Could you check a few things on this model? Use its own coordinates, in mm. Round coordinates to 2 decimals unless told otherwise and drop trailing zeros. Order: outer loops, then holes, each group sorted by start corner. A loop starts at its lowest first (then second) coordinate and runs counter-clockwise, first axis right, second up. Notation, with made-up numbers: (-32.5, 7) -> (19.5, 7) arc R30 cw to (19.5, 37) -> close; hole circle Ø10 at (58, 42.5). An arc over 180 degrees is marked (long way). One line per question, with ' | ' between items.
```python
from build123d import *

# Parameters (mm, degrees)
F0_W     = 32.5
F0_H     = 4
F0_W_2   = 15
F1_DEPTH = 4


with BuildPart() as f1:
    # F0 (on Top) → F1 (new body)
    with BuildSketch(Plane.XY):
        Polygon((0, -16), (0, 0), (-148, 0), (-148, -16), (-148, -20), (-148, -36), (0, -36), (0, -20), align=None)
        with Locations((-127.75, -18)):
            Rectangle(F0_W, F0_H, mode=Mode.SUBTRACT)
        with Locations((-89, -18)):
            Rectangle(F0_W_2, F0_H, mode=Mode.SUBTRACT)
        with Locations((-59, -18)):
            Rectangle(F0_W_2, F0_H, mode=Mode.SUBTRACT)
        with Locations((-20.25, -18)):
            Rectangle(F0_W, F0_H, mode=Mode.SUBTRACT)
    extrude(amount=F1_DEPTH)


solid = f1.part
```
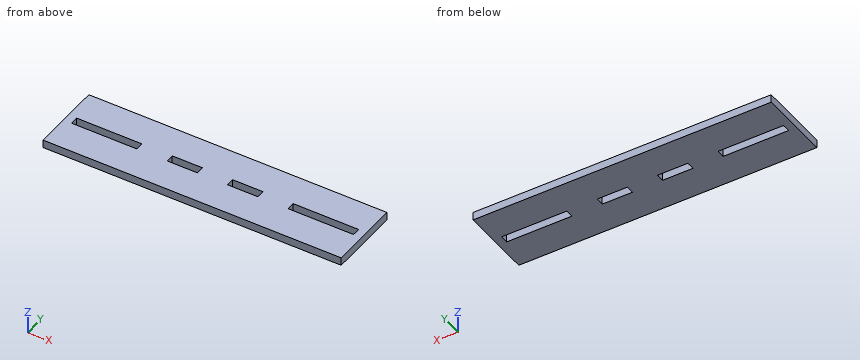
1. I need wall thicknesses on probe 1 along Y at (x, z) = (-131, 2.8); probe 2 along X at (y, z) = (-18, 1.5). Which ranges of each line are inside material? Lowest first, please.
From the geometry:
probe 1: y = -36 to -20, -16 to 0 | probe 2: x = -148 to -144, -111.5 to -96.5, -81.5 to -66.5, -51.5 to -36.5, -4 to 0
2. I want a section at B-B on y = -17.5. List the corners of the cut face in (x, z) for me, and give its area (3 significant figures).
From the geometry:
outline: (-148, 0) -> (-144, 0) -> (-144, 4) -> (-148, 4) -> close; (-111.5, 0) -> (-96.5, 0) -> (-96.5, 4) -> (-111.5, 4) -> close; (-81.5, 0) -> (-66.5, 0) -> (-66.5, 4) -> (-81.5, 4) -> close; (-51.5, 0) -> (-36.5, 0) -> (-36.5, 4) -> (-51.5, 4) -> close; (-4, 0) -> (0, 0) -> (0, 4) -> (-4, 4) -> close | area: 212 mm²
3. I want a section at A-A on x = -132. List the corners of the cut face in (y, z) for me.
From the geometry:
outline: (-36, 0) -> (-20, 0) -> (-20, 4) -> (-36, 4) -> close; (-16, 0) -> (0, 0) -> (0, 4) -> (-16, 4) -> close
4. I want a section at C-C on z = 1.05. List the corners of the cut face in (x, y) for me, and give its area (3 significant figures).
From the geometry:
outline: (-148, -36) -> (0, -36) -> (0, 0) -> (-148, 0) -> close; hole (-144, -20) -> (-111.5, -20) -> (-111.5, -16) -> (-144, -16) -> close; hole (-96.5, -20) -> (-81.5, -20) -> (-81.5, -16) -> (-96.5, -16) -> close; hole (-66.5, -20) -> (-51.5, -20) -> (-51.5, -16) -> (-66.5, -16) -> close; hole (-36.5, -20) -> (-4, -20) -> (-4, -16) -> (-36.5, -16) -> close | area: 4,950 mm²
